Autodesk Fusion 360 part; units mm, degrees
sketch "Sketch1" plane through (0, 0, 0) normal (0, 0, 1) x (1, 0, 0)
  circle A0 centre (0, 0) radius 22.25
  line L0 (0, 0) -> (0, 22.25) construction
  circle A1 centre (0, 17.75) radius 2.5
  line L1 (0, 17.75) -> (0, 20.25) construction
  circle A2 centre (-15.372, -8.875) radius 2.5
  circle A3 centre (15.372, -8.875) radius 2.5
  circle A4 centre (0, 0) radius 17.75 construction
  dimension "d1" = 44.5
  dimension "d2" = 5
  dimension "d3" = 2
  dimension "d5" = 360
extrude "Extrude1" add sketch "Sketch1" along normal blind 2.5 makes body 1
sketch "Sketch2" plane through (0, 0, 2.5) normal (0, 0, 1) x (-1, 0, 0)
  circle A0 centre (0, -17.75) radius 2.5
  circle A1 centre (15.372, 8.875) radius 2.5
  circle A2 centre (-15.372, 8.875) radius 2.5
  circle A3 centre (0, 0) radius 22.25
  circle A4 centre (0, 0) radius 11
  dimension "d8" = 22
extrude "Extrude2" add sketch "Sketch2" along normal blind 6.7 contours A4 bodies 1
sketch "Sketch3" plane through (0, 0, 9.2) normal (0, 0, 1) x (-1, 0, 0)
  circle A0 centre (0, 0) radius 11
  circle A1 centre (0, 0) radius 5
  dimension "d11" = 10
extrude "Extrude3" add sketch "Sketch3" along normal blind 5.5 contours A1 bodies 1
sketch "Sketch4" plane through (0, 0, 0) normal (0, 0, -1) x (1, 0, 0)
  circle A0 centre (0, -17.75) radius 2.5
  circle A1 centre (-15.372, 8.875) radius 2.5
  circle A2 centre (15.372, 8.875) radius 2.5
  circle A3 centre (0, 0) radius 22.25
  circle A4 centre (0, 0) radius 11
  dimension "d14" = 22
extrude "Extrude4" add sketch "Sketch4" along normal blind 39 contours A4 bodies 1
copy_body "Body->Comp1" bodies 1 removing the originals makes body 2 in component "Component"
component "Component" placed x (1, 0, 0) y (0, 1, 0) z (0, 0, 1) at (0, 0, 0)
Read the model definition and answer for the solid it produces. Units are mm, in the model's axes. A direction names the side the tool comes from. Give positions to 0.01 mm unless a question says otherwise; leave off trailing zeros. Order: outer loops, then holes, each group sorted by start corner. A loop starts at its lowest first (then second) coordinate and runs counter-clockwise, first axis right, second up.
(1) Find section B-B (y = 0). Give the vertices of the cut face in (x, z), plus the area to 3 significant figures.
(2) Straight lines are drawn through the part: L1, parallel to Y at x = 0, z = 0.65; L2, parallel to Z at x = -11, y = -12; L3, parallel to Z at x = -2.5, y = 6.5. For each, find the intervals that lie inside material, in ascending order.
(3) Given pin 1 (6.5 mm diameter, centred on x = 15.372, y = -8.875, fed in from +Z); pin 2 (12 mm diameter, centred on y = -11.5, z = -29, fed in from +X); pin 3 (6 mm diameter, centred on x = -13, z = -0.5, fed in from +Y) (3 decimals); pin 4 (22 mm diameter, centred on x = -9, y = 6.5, fed in from -Z), each flat-ended and moving along its own axis, determine where each tip first touches the part or whether it passes through.
(4) For a pull along X with two mould halves and no side action, classify faces 1 (the flat face through (-10, -5, 2.5)), 2 (the cylindrical face through (-17.356, -7.354, 1.232)), 3 (the cylindrical face through (2.38, -10.74, 5.8)) as released by +X, released by -X, zero draft, split by the parting line, or undercut.
(5) Find section D-D (z = -27). Give the vertices of the cut face in (x, y).
(6) Find section A-A (x = 0). Give the vertices of the cut face in (y, z), plus the area to 3 significant figures.
(7) Find section C-C (y = 17.75). Give the vertices of the cut face in (x, z), plus the area to 3 significant figures.
(8) For faces 4 (the flat face through (-10, -5, 0)), 5 (the cylindrical face through (17.681, -7.917, 1.232)), 6 (the cylindrical face through (1.08, -4.88, 11.91)), determine the directions among +Z, -Z, +X, -X, +Y, -Y from which every point of the face is accessible in a straight line to the end or side of a thin tool.
Result sheet:
1. outline: (-22.25, 0) - (-11, 0) - (-11, -39) - (11, -39) - (11, 0) - (22.25, 0) - (22.25, 2.5) - (11, 2.5) - (11, 9.2) - (5, 9.2) - (5, 14.7) - (-5, 14.7) - (-5, 9.2) - (-11, 9.2) - (-11, 2.5) - (-22.25, 2.5) - close
1. area: 1,170 mm2
2. L1: y = -22.25 to 15.25, 20.25 to 22.25
2. L2: z = 0 to 2.5
2. L3: z = -39 to 9.2
3. pin 1: stops at z = 2.5
3. pin 2: stops at x = 9.53
3. pin 3: stops at y = 19.855
3. pin 4: stops at z = -39
4. face 1: zero draft
4. face 2: undercut
4. face 3: split by the parting line
5. outline: circle Ø22 at (0, 0)
6. outline: (-22.25, 0) - (-11, 0) - (-11, -39) - (11, -39) - (11, 0) - (15.25, 0) - (15.25, 2.5) - (11, 2.5) - (11, 9.2) - (5, 9.2) - (5, 14.7) - (-5, 14.7) - (-5, 9.2) - (-11, 9.2) - (-11, 2.5) - (-22.25, 2.5) - close; (20.25, 0) - (22.25, 0) - (22.25, 2.5) - (20.25, 2.5) - close
6. area: 1,160 mm2
7. outline: (-13.42, 0) - (-2.5, 0) - (-2.5, 2.5) - (-13.42, 2.5) - close; (2.5, 0) - (13.42, 0) - (13.42, 2.5) - (2.5, 2.5) - close
7. area: 54.6 mm2
8. face 4: -Z
8. face 5: +Z, -Z
8. face 6: +Z
